```python
from build123d import *

# Parameters (mm, degrees)
EXTRUDE_1_DEPTH = 3


with BuildPart() as part:
    # 草图1 → 凸台-拉伸1 (new body)
    with BuildSketch(Plane.XY):
        Polygon((-25, -10), (-20, -10), (-20, -13), (-10, -13), (-10, -10), (-5, -10), (-5, -13), (5, -13), (5, -10), (10, -10), (10, -13), (20, -13), (20, -10), (25, -10), (25, -8), (28, -8), (28, -2), (25, -2), (25, 2), (28, 2), (28, 8), (25, 8), (25, 10), (20, 10), (20, 13), (10, 13), (10, 10), (5, 10), (5, 13), (-5, 13), (-5, 10), (-10, 10), (-10, 13), (-20, 13), (-20, 10), (-25, 10), (-25, 8), (-28, 8), (-28, 2), (-25, 2), (-25, -2), (-28, -2), (-28, -8), (-25, -8), align=None)
        Polygon((-12.5, 7), (12.5, 7), (0, 2), align=None, mode=Mode.SUBTRACT)
        Polygon((20, 5), (20, -5), (7.08425002, 0), align=None, mode=Mode.SUBTRACT)
        Polygon((-20, 5), (-7.08425002, 0), (-20, -5), align=None, mode=Mode.SUBTRACT)
        Polygon((-12.5, -7), (0, -2), (12.5, -7), align=None, mode=Mode.SUBTRACT)
    extrude(amount=EXTRUDE_1_DEPTH)


solid = part.part
```
Design review of the part built by this model. Coordinates are the model's own, in mm. A direction names the side the tool comes from. Give positions to 0.01 mm unless a question says otherwise; leave off trailing zeros. Order: outer loops, then holes, each group sorted by start corner. A loop starts at its lowest first (then second) coordinate and runs counter-clockwise, first axis right, second up. Notation, with made-up numbers: (3, 36) -> (35, 36) arc R31 cw to (35, 75) -> close; hole circle Ø7 at (47, 68). An arc over 180 degrees is marked (long way). Write each question's results on one line, items separated by ' | '. Start each with the question number.
Q1. Machinability: for faces 1 (the flat face through (5, -12, 1)), 2 (the flat face through (-20, 12, 1)), 3 (the flat face through (25, 9, 1)), 4 (the flat face through (-10, 11, 1)), 5 (the flat face through (-13.452, -2.465, 1.479)), which of the approach directions +Z, -Z, +X, -X, +Y, -Y give a long, thin tool a straight path to every point of the face, cutting with its end or side? Answer none if there is none.
Q2. Add section A-A on x = -6.5. Give the boundary of the cut face in (y, z), and give its area (3 significant figures).
Q3. Mouldability with a two-part tool opening along Y and no side actions: class faces 6 (the flat face through (-26, 8, 1)), 7 (the flat face through (6.337, 4.535, 1.479)), 8 (the flat face through (-10, -12, 1)) as +Y half, -Y half, draft (parallel to the pull), parting line (faces both ways), or undercut.
Q4. Add section D-D on y = -1. Give the boundary of the cut face in (x, z), and give its area (3 significant figures).
Q5. Wall thickness on L1, parallel to X at y = 10.5, z = 2.3; L2, parallel to Y at x = -6, z = 0.4; L3, parallel to Y at x = 9.5, z = 2.55: over which ranges is each line inside the solid? List them lowest first. Write a range as from..to.
Q6. For pin 1 (12 mm diameter, centred on x = 9.5, y = -1, fed in from -Z); pin 2 (0.9 mm diameter, centred on y = 11, z = 1, fed in from +X); pin 3 (1.5 mm diameter, centred on x = 26, z = 1.5, fed in from +Y); pin 4 (1.5 mm diameter, centred on x = -26, z = 2, fed in from -Y), all flat-tipped, find the tip position at first contact; note any pin that passes through.
Q7. Add section B-B on y = -4.25. Give the boundary of the cut face in (x, z) (3 decimals), and give its area (3 significant figures).
Q8. Add section C-C on x = -18.5. Give the boundary of the cut face in (y, z).
Found:
1) face 1: +Z, -Z, -Y | face 2: +Z, -Z, -X, +Y | face 3: +Z, -Z, +X, +Y | face 4: +Z, -Z, +Y | face 5: +Z, -Z
2) outline: (-10, 0) -> (-7, 0) -> (-7, 3) -> (-10, 3) -> close; (-4.6, 0) -> (4.6, 0) -> (4.6, 3) -> (-4.6, 3) -> close; (7, 0) -> (10, 0) -> (10, 3) -> (7, 3) -> close | area: 45.6 mm2
3) face 6: +Y half | face 7: undercut | face 8: draft
4) outline: (-25, 0) -> (-20, 0) -> (-20, 3) -> (-25, 3) -> close; (-9.67, 0) -> (9.67, 0) -> (9.67, 3) -> (-9.67, 3) -> close; (20, 0) -> (25, 0) -> (25, 3) -> (20, 3) -> close | area: 88.0 mm2
5) L1: x = -20..-10, -5..5, 10..20 | L2: y = -10..-7, -4.4..4.4, 7..10 | L3: y = -10..-7, -5.8..-0.94, 0.94..5.8, 7..10
6) pin 1: stops at z = 0 | pin 2: stops at x = 20 | pin 3: stops at y = 8 | pin 4: stops at y = -8
7) outline: (-28, 0) -> (-20, 0) -> (-20, 3) -> (-28, 3) -> close; (-18.063, 0) -> (-5.625, 0) -> (-5.625, 3) -> (-18.063, 3) -> close; (5.625, 0) -> (18.063, 0) -> (18.063, 3) -> (5.625, 3) -> close; (20, 0) -> (28, 0) -> (28, 3) -> (20, 3) -> close | area: 123 mm2
8) outline: (-13, 0) -> (-4.42, 0) -> (-4.42, 3) -> (-13, 3) -> close; (4.42, 0) -> (13, 0) -> (13, 3) -> (4.42, 3) -> close
